Geometry: final body of the model. Coordinates: model frame, mm. Face numbers are marked on the shaded views. A direction names the side the tool comes from. Coordinates: 2 decimals unless noted, no trailing zeros. Write each loop counter-clockwise with the first axis right and the second up, starting at its lowest first coordinate (ties: lowest second). Pieces come first, ordered by that corner, then holes.
from build123d import *

# Parameters (mm, degrees)
BOSS_EXTRUDE1_DEPTH        = 4
CUT_EXTRUDE1_DEPTH         = 3.75
CUT_EXTRUDE1_DEPTH_BACK    = 3.75
SKETCH2_R                  = 5.5
F_1_0MM_DOWEL_HOLE1_REACH  = 12.691
F_1_0MM_DOWEL_HOLE1_BORE_R = 0.205
LPATTERN1_COUNT            = 4
LPATTERN1_PITCH            = 2
MIRROR1_COPY_1_REACH       = 12.691
MIRROR1_COPY_1_SKETCH_R    = 0.205
MIRROR1_COPY_2_REACH       = 12.691
MIRROR1_COPY_2_SKETCH_R    = 0.205
MIRROR1_COPY_3_REACH       = 12.691
MIRROR1_COPY_3_SKETCH_R    = 0.205


with BuildPart() as part:
    # Sketch1 → Boss-Extrude1 (new, symmetric)
    with BuildSketch(Plane.XY):
        with BuildLine():
            Line((-1.5, 0), (-7.485975276, 0))
            Line((-7.485975276, 0), (-7.485975276, -0.41))
            Line((-7.485975276, -0.41), (-5.985975276, -0.41))
            ThreePointArc((-5.985975276, -0.41), (-5.186676874, -3.016352599), (-3.31662479, -5))
            Line((-3.31662479, -5), (-7, -5))
            Line((-7, -5), (-7, -6.5))
            Line((-7, -6.5), (7, -6.5))
            Line((7, -6.5), (7, -5))
            Line((7, -5), (3.31662479, -5))
            ThreePointArc((3.31662479, -5), (5.186676874, -3.016352599), (5.985975276, -0.41))
            Line((5.985975276, -0.41), (7.485975276, -0.41))
            Line((7.485975276, -0.41), (7.485975276, 0))
            Line((7.485975276, 0), (1.5, 0))
            ThreePointArc((1.5, 0), (0, -1.5), (-1.5, 0))
        make_face()
    extrude(amount=BOSS_EXTRUDE1_DEPTH, both=True)

    # Sketch2 → Cut-Extrude1 (cut, two sides: drawn at the far end of the back side and taken through both)
    with BuildSketch(Plane.XY.offset(-CUT_EXTRUDE1_DEPTH_BACK)):
        Circle(SKETCH2_R)
    extrude(amount=CUT_EXTRUDE1_DEPTH + CUT_EXTRUDE1_DEPTH_BACK, mode=Mode.SUBTRACT)

    # Ø1.0mm Dowel Hole1 bore → Ø1.0mm Dowel Hole1 (cut, up to next)
    with BuildSketch(Plane(origin=(0, 0, 0), x_dir=(1, 0, 0), z_dir=(0, 1, 0)), mode=Mode.PRIVATE) as f_1_0mm_dowel_hole1_sk1:
        with Locations((6.735975276, 3)):
            Circle(F_1_0MM_DOWEL_HOLE1_BORE_R)
    f_1_0mm_dowel_hole1_tool1 = extrude(f_1_0mm_dowel_hole1_sk1.sketch, amount=-F_1_0MM_DOWEL_HOLE1_REACH, mode=Mode.PRIVATE) & part.part
    f_1_0mm_dowel_hole1 = f_1_0mm_dowel_hole1_tool1.solids().sort_by_distance((6.735975, 0, -3))[0]
    add(f_1_0mm_dowel_hole1, mode=Mode.SUBTRACT)

    # LPattern1: Ø1.0mm Dowel Hole1 ×4
    with Locations(*[(0, 0, i * LPATTERN1_PITCH) for i in range(1, LPATTERN1_COUNT)]):
        add(f_1_0mm_dowel_hole1, mode=Mode.SUBTRACT)

    # Mirror1: Ø1.0mm Dowel Hole1 across plane
    add(f_1_0mm_dowel_hole1.mirror(Plane(origin=(0, 0, 0), x_dir=(0, 0, 1), z_dir=(1, 0, 0))), mode=Mode.SUBTRACT)

    # Mirror1 copy 1 sketch → Mirror1 copy 1 (cut, up to next)
    with BuildSketch(Plane(origin=(0, 0, 2), x_dir=(-1, 0, 0), z_dir=(0, 1, 0)), mode=Mode.PRIVATE) as mirror1_copy_1_sk1:
        with Locations((6.735975276, -3)):
            Circle(MIRROR1_COPY_1_SKETCH_R)
    mirror1_copy_1_tool1 = extrude(mirror1_copy_1_sk1.sketch, amount=-MIRROR1_COPY_1_REACH, mode=Mode.PRIVATE) & part.part
    add(mirror1_copy_1_tool1.solids().sort_by_distance((-6.735975, 0, -1))[0], mode=Mode.SUBTRACT)

    # Mirror1 copy 2 sketch → Mirror1 copy 2 (cut, up to next)
    with BuildSketch(Plane(origin=(0, 0, 4), x_dir=(-1, 0, 0), z_dir=(0, 1, 0)), mode=Mode.PRIVATE) as mirror1_copy_2_sk1:
        with Locations((6.735975276, -3)):
            Circle(MIRROR1_COPY_2_SKETCH_R)
    mirror1_copy_2_tool1 = extrude(mirror1_copy_2_sk1.sketch, amount=-MIRROR1_COPY_2_REACH, mode=Mode.PRIVATE) & part.part
    add(mirror1_copy_2_tool1.solids().sort_by_distance((-6.735975, 0, 1))[0], mode=Mode.SUBTRACT)

    # Mirror1 copy 3 sketch → Mirror1 copy 3 (cut, up to next)
    with BuildSketch(Plane(origin=(0, 0, 6), x_dir=(-1, 0, 0), z_dir=(0, 1, 0)), mode=Mode.PRIVATE) as mirror1_copy_3_sk1:
        with Locations((6.735975276, -3)):
            Circle(MIRROR1_COPY_3_SKETCH_R)
    mirror1_copy_3_tool1 = extrude(mirror1_copy_3_sk1.sketch, amount=-MIRROR1_COPY_3_REACH, mode=Mode.PRIVATE) & part.part
    add(mirror1_copy_3_tool1.solids().sort_by_distance((-6.735975, 0, 3))[0], mode=Mode.SUBTRACT)


solid = part.part
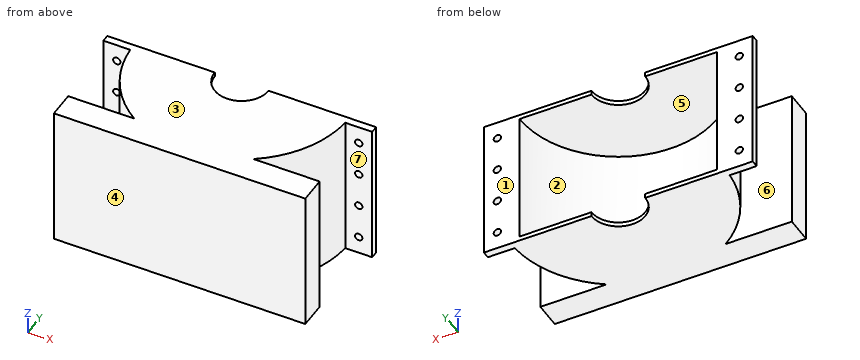
Item 1: Section A-A, the plane z = -1. Output: boundary loops of the cut face in (x, y), plus the area to 3 significant figures.
Derived:
outline: (-7.49, -0.41) - (-6.94, -0.41) - (-6.94, 0) - (-7.49, 0) - close; (-7, -6.5) - (7, -6.5) - (7, -5) - (3.32, -5) arc R6 ccw to (5.99, -0.41) - (6.53, -0.41) - (6.53, 0) - (5.5, 0) arc R5.5 cw to (-5.5, 0) - (-6.53, 0) - (-6.53, -0.41) - (-5.99, -0.41) arc R6 ccw to (-3.32, -5) - (-7, -5) - close; (6.94, -0.41) - (7.49, -0.41) - (7.49, 0) - (6.94, 0) - close
area: 26.4 mm2
Item 2: Material intervals for probe 1 along Z at (x, y) = (-2, -0.75); probe 2 along X at (y, z) = (-0.15, -3); probe 3 along Y at (x, z) = (-4.5, -1), sorted ascending.
Derived:
probe 1: z = -4 to -3.75, 3.75 to 4
probe 2: x = -7.49 to -6.94, -6.53 to -5.5, 5.5 to 6.53, 6.94 to 7.49
probe 3: y = -6.5 to -5, -3.97 to -3.16
Item 3: Pin query (flat end, axial travel): pin 1 (3 mm diameter, centred on x = -5, z = -1.5, fed in from +Y); pin 2 (1.6 mm diameter, centred on y = -6, z = 1.5, fed in from -X); pin 3 (0.8 mm diameter, centred on y = -5.5, z = 0.5, fed in from +X); pin 4 (2 mm diameter, centred on y = -3.5, z = 3, fed in from +X). Return the tip coordinate at first contact, or that it passes through.
Derived:
pin 1: stops at y = 0
pin 2: stops at x = -7
pin 3: stops at x = 7
pin 4: stops at x = 5.45
Item 4: Section B-B, the plane x = 0. Output: boundary loops of the cut face in (y, z), plus the area to 3 significant figures.
Derived:
outline: (-6.5, -4) - (-1.5, -4) - (-1.5, -3.75) - (-5.5, -3.75) - (-5.5, 3.75) - (-1.5, 3.75) - (-1.5, 4) - (-6.5, 4) - close
area: 10.0 mm2
Item 5: Section D-D, the plane x = 5. Output: boundary loops of the cut face in (y, z).
Derived:
outline: (-6.5, -4) - (-5, -4) - (-5, 4) - (-6.5, 4) - close; (-3.32, -4) - (0, -4) - (0, -3.75) - (-2.29, -3.75) - (-2.29, 3.75) - (0, 3.75) - (0, 4) - (-3.32, 4) - close
Item 6: Section C-C, the plane y = -3.5. Output: boundary loops of the cut face in (x, z), plus the area to 3 significant figures.
Derived:
outline: (-4.87, -4) - (4.87, -4) - (4.87, 4) - (-4.87, 4) - close; hole (-4.24, -3.75) - (4.24, -3.75) - (4.24, 3.75) - (-4.24, 3.75) - close
area: 14.3 mm2
Item 7: Set-up query: the marked faces 3, 4, 5, 6 and 7. Return all of +Z, -Z, +X, -X, +Y, -Y with unobstructed straight access to the full face (end or side cutting, diameter ignored); none if empty.
Derived:
face 3: +Z, +X, -X, +Y, -Y
face 4: +Z, -Z, +X, -X, -Y
face 5: +Y
face 6: +Z, -Z, -X
face 7: +Z, -Z, +X
Item 8: Pull-direction query (X, two-part tool) for the marked faces 1 and 2; classes: released by +X, released by -X, zero draft, split by the parting line, or undercut.
Derived:
face 1: zero draft
face 2: undercut
